Can you work these out from the model? Positions are in its coordinate system, mm. Coordinates: 2 decimals unless noted, no trailing zeros. Order: outer loops, then holes, each group sorted by start corner. A loop starts at its lowest first (then second) coordinate and runs counter-clockwise, first axis right, second up. Notation, with made-up numbers: (-2.75, 4.5) - (9.25, 4.5) arc R22 ccw to (9.25, 24.5) - close; hole circle Ø7 at (-6, 43). An arc over 180 degrees is marked (long way). Return JSON: item names as keys, results as strings. Group by question number.
1) If I drill on line 1 along Y through (x, z) = (-63, -1.35); line 2 along Y through (x, z) = (64.5, -0.4); line 3 along Y through (x, z) = (46, -0.9), over which ranges is the centre line in solid material (lowest first)?
2) For pin 1 Ø2.5 at (x, y) = (-63.32, 8.27) entering from +Z, with a flat end and sliding along its axis, tell me the tip position at first contact or that it passes through.
3) Imagine slicing it at B-B (z = -1). Write out the boundary of the cut face in (x, y) (3 decimals), and give its area (3 significant figures).
4) Imagine slicing it at A-A (x = 45). Write out the boundary of the cut face in (y, z), and give its area (3 significant figures).
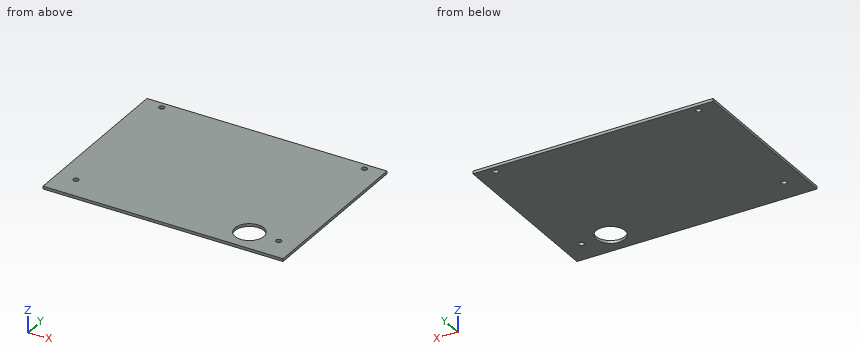
```python
from build123d import *

# Parameters (mm, degrees)
SKETCH1_W            = 150
SKETCH1_H            = 108.5
BASE_FLANGE1_DEPTH   = 1.75
CUT_EXTRUDE1_REACH   = 128.436
SKETCH6_R            = 9
M3_CLEARANCE_HOLE1_D = 3.4


# Sheet-metal steps are written as plain solids
with BuildPart() as part:
    # Sketch1 → Base-Flange1 (new body)
    with BuildSketch(Plane.XY):
        with Locations((0, 47.52414015)):
            Rectangle(SKETCH1_W, SKETCH1_H)
    extrude(amount=-BASE_FLANGE1_DEPTH)

    # Sketch6 → Cut-Extrude1 (cut, up to next)
    with BuildSketch(Plane.XY, mode=Mode.PRIVATE) as cut_extrude1_sk1:
        with Locations((45, 8.27414015)):
            Circle(SKETCH6_R)
    cut_extrude1_tool1 = extrude(cut_extrude1_sk1.sketch, amount=-CUT_EXTRUDE1_REACH, mode=Mode.PRIVATE) & part.part
    add(cut_extrude1_tool1.solids().sort_by_distance((45, 8.27414, 0))[0], mode=Mode.SUBTRACT)

    # M3 Clearance Hole1 (through all)
    with Locations(Plane.XY):
        with Locations((63.325, 8.27414015), (63.325, 97.64914015)):
            m3_clearance_hole1 = Hole(M3_CLEARANCE_HOLE1_D / 2)

    # Mirror1: M3 Clearance Hole1 across plane
    add(m3_clearance_hole1.mirror(Plane(origin=(0, 0, 0), x_dir=(0, 0, 1), z_dir=(1, 0, 0))), mode=Mode.SUBTRACT)


solid = part.part
```
Calculated:
{
 "1": {"line 1": "-6.73 to 6.61, 9.94 to 95.98, 99.32 to 101.77", "line 2": "-6.73 to 7.05, 9.5 to 96.42, 98.88 to 101.77", "line 3": "-6.73 to -0.67, 17.22 to 101.77"},
 "2": {"pin 1": "through"},
 "3": {"outline": "(-75, -6.726) - (75, -6.726) - (75, 101.774) - (-75, 101.774) - close; hole circle Ø3.4 at (-63.325, 8.274); hole circle Ø3.4 at (-63.325, 97.649); hole circle Ø18 at (45, 8.274); hole circle Ø3.4 at (63.325, 8.274); hole circle Ø3.4 at (63.325, 97.649)", "area": "16,000 mm2"},
 "4": {"outline": "(-6.73, -1.75) - (-0.73, -1.75) - (-0.73, 0) - (-6.73, 0) - close; (17.27, -1.75) - (101.77, -1.75) - (101.77, 0) - (17.27, 0) - close", "area": "158 mm2"}
}
